Autodesk Fusion 360 part; units mm, degrees
sketch "Sketch1" plane through (0, 0, 0) normal (0, 0, 1) x (1, 0, 0)
  line L0 (0, 0) -> (20, 0)
  line L1 (20, 0) -> (20, 20)
  line L2 (20, 20) -> (0, 20)
  line L3 (0, 20) -> (0, 0)
  circle A0 centre (10, 10) radius 7.5
  dimension "d1" = 20
  dimension "d2" = 20
  dimension "d3" = 15
extrude "Extrude1" add sketch "Sketch1" along normal blind 20
extrude "Extrude2" add sketch "Sketch1" along normal blind 2 contours A0
sketch "Sketch2" plane through (0, 0, 0) normal (1, 0, 0) x (0, 1, 0)
  circle A0 centre (10, 10) radius 5
  dimension "d9" = 10
extrude "Extrude3" cut sketch "Sketch2" along normal blind 20 and the other way blind 0
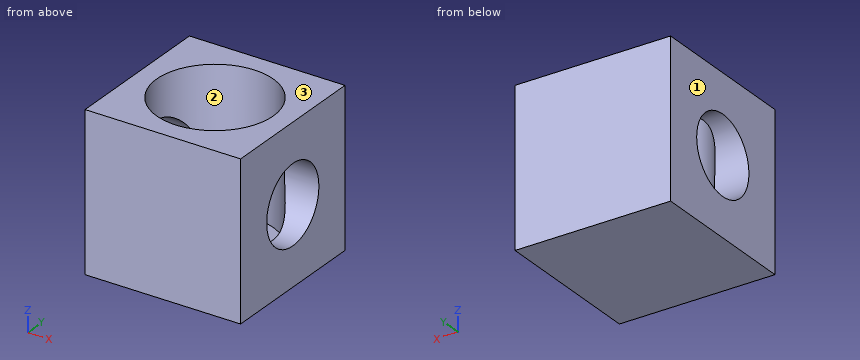
The listing builds one solid part. Answer for the finished solid, in the listing's coordinates (mm). Face numbers are marked on the shaded views. Round coordinates to 2 decimals unless told otherwise and drop trailing zeros. Loops run counter-clockwise (first coordinate to the right, second up) from the corner with the lowest first, then second, coordinate; pieces in that order, holes last.
Q1. For a pull along X with two mould halves and no side action, classify the marked faces 1, 2 and 3 as released by +X, released by -X, zero draft, split by the parting line, or undercut.
Q2. Section A-A, the plane y = 10 is taken. Determine the outline of the cut face in (x, z).
Q3. Given pin 1 Ø9 at (y, z) = (10, 10) entering from -X; pin 2 Ø4 at (y, z) = (7.5, 13) entering from +X; pin 3 Ø7.5 at (x, y) = (9, 8) entering from +Z, each flat-ended and moving along its own axis, determine where each tip first touches the part or whether it passes through.
Q4. Find the intervals of material crossed by line 1 (Y direction, x = 1.75, z = 10); line 2 (Y direction, x = 5, z = 3.75); line 3 (Z direction, x = 17, y = 11.25), in increasing order.
Q5. Section B-B, the plane x = 10 is taken. Determine the outline of the cut face in (y, z), then the cut area to 3 significant figures.
Q6. Section C-C, the plane z = 10 is taken. Determine the outline of the cut face in (x, y).
Q7. Section D-D, the plane z = 2.5 is taken. Determine the outline of the cut face in (x, y).
Completed:
1. face 1: released by -X
1. face 2: undercut
1. face 3: zero draft
2. outline: (0, 0) - (20, 0) - (20, 5) - (17.5, 5) - (17.5, 2) - (2.5, 2) - (2.5, 5) - (0, 5) - close; (0, 15) - (2.5, 15) - (2.5, 20) - (0, 20) - close; (17.5, 15) - (20, 15) - (20, 20) - (17.5, 20) - close
3. pin 1: passes through
3. pin 2: stops at x = 20
3. pin 3: stops at z = 2
4. line 1: y = 0 to 5, 15 to 20
4. line 2: y = 0 to 4.41, 15.59 to 20
4. line 3: z = 0 to 2
5. outline: (0, 0) - (20, 0) - (20, 20) - (17.5, 20) - (17.5, 2) - (2.5, 2) - (2.5, 20) - (0, 20) - close
5. area: 130 mm2
6. outline: (0, 0) - (20, 0) - (20, 5) - (15.59, 5) arc R7.5 cw to (4.41, 5) - (0, 5) - close; (0, 15) - (4.41, 15) arc R7.5 cw to (15.59, 15) - (20, 15) - (20, 20) - (0, 20) - close
7. outline: (0, 0) - (20, 0) - (20, 20) - (0, 20) - close; hole circle Ø15 at (10, 10)
